Could you check a few things on this drawing? It's one solid part, dimensions in mm from its lowest x, y, z. Round coordinates to 2 decimals unless told otherwise and drop trailing zeros. Write each loop counter-clockwise with the first axis right and the second up, starting at its lowest first coordinate (ties: lowest second). Pieces come first, ordered by that corner, then holes. Notation, with made-up numbers: (85.5, 60.25) -> (126.5, 60.25) arc R18 ccw to (126.5, 87.25) -> close; hole circle Ø9 at (89, 62). An arc over 180 degrees is marked (long way). Answer in a Markdown table with one row per item.
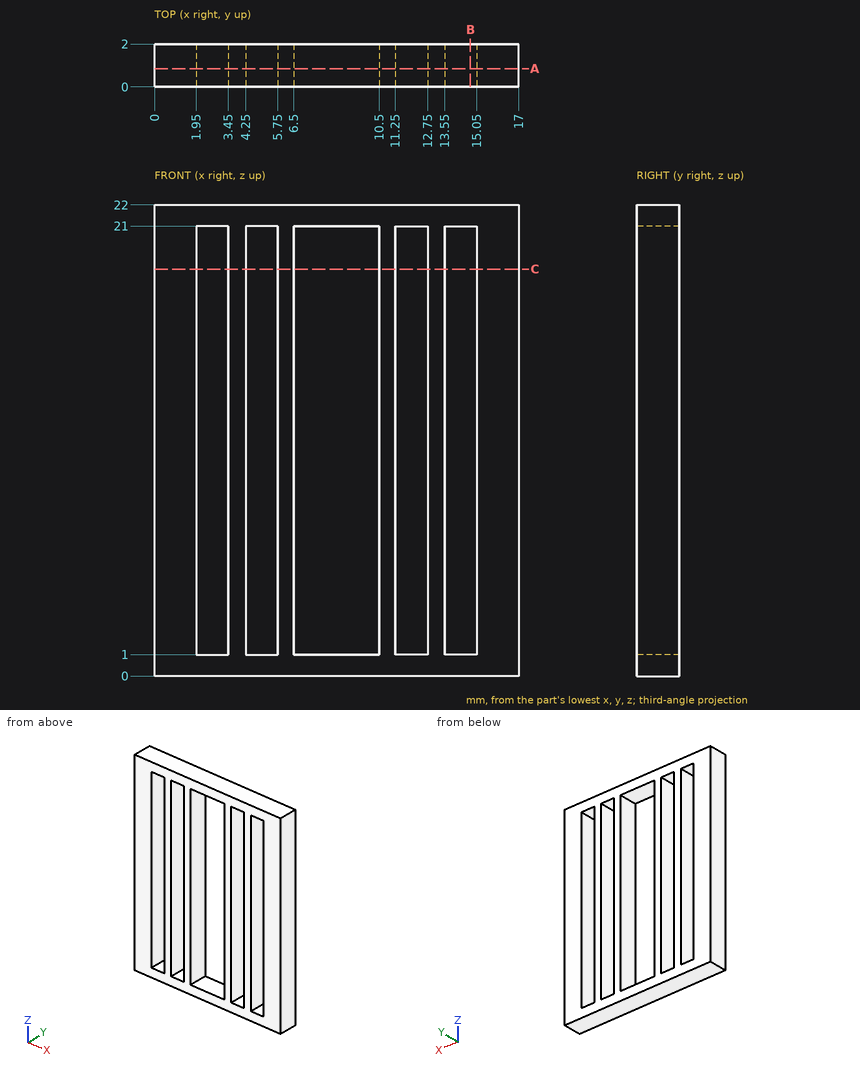
1) I want a section at C-C, the plane z = 19. List the corners of the cut face in (x, y) for me, and give its area (3 significant figures).
Response:
| item | result |
|---|---|
| outline | (0, 0) -> (1.95, 0) -> (1.95, 2) -> (0, 2) -> close; (3.45, 0) -> (4.25, 0) -> (4.25, 2) -> (3.45, 2) -> close; (5.75, 0) -> (6.5, 0) -> (6.5, 2) -> (5.75, 2) -> close; (10.5, 0) -> (11.25, 0) -> (11.25, 2) -> (10.5, 2) -> close; (12.75, 0) -> (13.55, 0) -> (13.55, 2) -> (12.75, 2) -> close; (15.05, 0) -> (17, 0) -> (17, 2) -> (15.05, 2) -> close |
| area | 14.0 mm^2 |
2) I want a section at A-A, the plane y = 0.85. List the corners of the cut face in (x, z) for me, and give its area (3 significant figures).
Response:
| item | result |
|---|---|
| outline | (0, 0) -> (17, 0) -> (17, 22) -> (0, 22) -> close; hole (1.95, 1) -> (3.45, 1) -> (3.45, 21) -> (1.95, 21) -> close; hole (4.25, 1) -> (5.75, 1) -> (5.75, 21) -> (4.25, 21) -> close; hole (6.5, 1) -> (10.5, 1) -> (10.5, 21) -> (6.5, 21) -> close; hole (11.25, 1) -> (12.75, 1) -> (12.75, 21) -> (11.25, 21) -> close; hole (13.55, 1) -> (15.05, 1) -> (15.05, 21) -> (13.55, 21) -> close |
| area | 174 mm^2 |
3) I want a section at B-B, the plane x = 14.75. List the corners of the cut face in (y, z) for me, and give its area (3 significant figures).
Response:
| item | result |
|---|---|
| outline | (0, 0) -> (2, 0) -> (2, 1) -> (0, 1) -> close; (0, 21) -> (2, 21) -> (2, 22) -> (0, 22) -> close |
| area | 4.00 mm^2 |
4) I need wall thicknesses on line 1 (X direction, y = 0.95, z = 6); line 2 (Z direction, x = 14.5, y = 0.95). Which ranges of each line are inside material? Lowest first, please. Write a range as [from, to].
Response:
| item | result |
|---|---|
| line 1 | x = [0, 1.95], [3.45, 4.25], [5.75, 6.5], [10.5, 11.25], [12.75, 13.55], [15.05, 17] |
| line 2 | z = [0, 1], [21, 22] |
